Geometry: final body of the model. Coordinates: model frame, mm. Face numbers are marked on the shaded views. A direction names the side the tool comes from. Round coordinates to 2 decimals unless told otherwise and drop trailing zeros. Write each loop counter-clockwise with the first axis right and the second up, starting at its lowest first coordinate (ties: lowest second). Pieces come first, ordered by that corner, then holes.
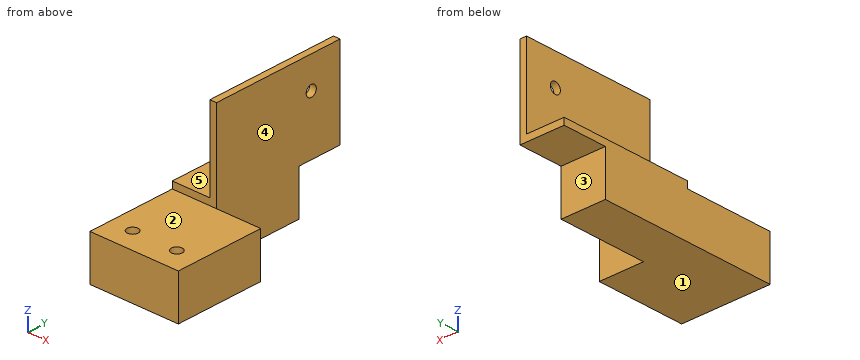
Autodesk Inventor part; units mm, degrees
ref_plane "YZ Plane" through (0, 0, 0) normal (1, 0, 0) x (0, 1, 0)
ref_plane "XZ Plane" through (0, 0, 0) normal (0, 1, 0) x (-1, 0, 0)
ref_plane "XY Plane" through (0, 0, 0) normal (0, 0, 1) x (1, 0, 0)
sketch "Náčrt1" plane through (0, 0, 0) normal (0, 0, 1) x (1, 0, 0)
  line L0 (-14, 0) -> (14, 0)
  line L1 (0, 28) -> (0, -28)
  line L2 (-10, 20) -> (10, 20)
  line L3 (10, 20) -> (10, -20)
  line L4 (10, -20) -> (-10, -20)
  line L5 (-10, -20) -> (-10, 20)
  point P0 (0, 0)
  dimension "d0" = 20
  dimension "d1" = 40
extrude "Vysunutí1" add sketch "Náčrt1" along normal mid plane 10
sketch "Náčrt2" plane through (0, 0, 5) normal (0, 0, 1) x (1, 0, 0)
  line L0 (-10, -20) -> (10, -20)
  line L1 (10, -20) -> (10, 20)
  line L2 (10, 20) -> (-10, 20)
  line L3 (-10, 20) -> (-10, -20)
  line L4 (10, -20) -> (10, 20)
  line L5 (0, 20) -> (10, 20)
  line L6 (10, 20) -> (10, 0)
  line L7 (10, 0) -> (0, 0)
  line L8 (0, 0) -> (0, 20)
  point P0 (0, 0)
extrude "Vysunutí2" cut sketch "Náčrt2" against normal through all contours L7 L8 L2 L1
sketch "Náčrt3" plane through (0, 0, 5) normal (0, 0, 1) x (1, 0, 0)
  line L0 (10, -20) -> (10, 0)
  line L1 (-10, -20) -> (10, -20)
  point P0 (0, 0)
  point P1 (-5, -15)
  point P2 (5, -15)
  dimension "d6" = 5
  dimension "d7" = 10
  dimension "d8" = 5
  dimension "d9" = 5
hole "Díra1" at (-5, -15, 5) at (5, -15, 5) direction (0, 0, -1) diameter 2.459 depth 5
sketch "Náčrt4" plane through (0, 0, 5) normal (0, 0, 1) x (1, 0, 0)
  line L0 (0, 0) -> (-10, 0)
  line L1 (-10, 0) -> (-10, 30)
  line L2 (-10, 30) -> (0, 30)
  line L3 (0, 30) -> (0, 0)
  dimension "d17" = 10
  dimension "d18" = 30
extrude "Vysunutí3" add sketch "Náčrt4" along normal blind 20
sketch "Náčrt5" plane through (-10, 30, 5) normal (0, 1, 0) x (1, 0, 0)
  line L0 (0, -20) -> (10, -20)
  line L1 (0, -20) -> (8.5, -20)
  line L2 (8.5, -20) -> (8.5, -1.5)
  line L3 (8.5, -1.5) -> (0, -1.5)
  line L4 (0, -1.5) -> (0, -20)
  point P0 (10, 5)
  dimension "d21" = 8.5
  dimension "d22" = 18.5
extrude "Vysunutí4" cut sketch "Náčrt5" against normal through all
sketch "Náčrt6" plane through (0, 0, -5) normal (1, 0, 0) x (0, 0, -1)
  line L0 (0, 20) -> (0, 0)
  line L1 (-10, 20) -> (0, 20)
  line L2 (-10, 20) -> (-10, 30)
  line L3 (-10, 30) -> (-30, 30)
  line L4 (-30, 0) -> (-30, 30)
  line L5 (-10, 0) -> (-30, 0)
  line L6 (-10, 0) -> (0, 0)
  point P0 (-5, 0)
  point P1 (-23, 23)
  dimension "d25" = 7
  dimension "d26" = 7
hole "Díra2" at (0, 23, 18) direction (-1, 0, 0) diameter 2.459 end through all
properties part number "x_bearing_tab" material "Hliník 6061"
1) Section B-B on x = -0.5. Output: boundary loops of the cut face in (y, z).
2) First-contact query: P1, Ø2.5, axis at x = -5.5, y = -15, coming from the +Z side; P2, Ø3, axis at x = -3.5, y = 24.5, coming from the -Z side; P3, Ø3, axis at y = 23, z = 18, coming from the +X side. Flat tips, straight axial feed; report the tip coordinate or a pass-through.
3) Reachability of the marked faces 1, 2, 3, 4 and 5 from +Z, -Z, +X, -X, +Y, -Y: full face, straight path, thin tool, end or side. Return the list, or none.
4) Line query: probe 1 along X at (y, z) = (-15, 3.7); probe 2 along Y at (x, z) = (-0.7, 18); probe 3 along Y at (x, z) = (5, 3.1). Output: solid intervals per line, ascending.
5) Section D-D on x = 5. Output: boundary loops of the cut face in (y, z).
6) Section C-C on z = 18. Output: boundary loops of the cut face in (x, y).
7) Section A-A on y = 23. Output: boundary loops of the cut face in (x, z).
Filled in:
1. outline: (-20, -5) - (20, -5) - (20, 5) - (30, 5) - (30, 25) - (0, 25) - (0, 5) - (-20, 5) - close; hole circle Ø2.46 at (23, 18)
2. P1: stops at z = 5
2. P2: stops at z = 5
2. P3: stops at x = 0
3. face 1: -Z, +X, -X, +Y, -Y
3. face 2: +Z, +X, -X, -Y
3. face 3: -Z, +X, -X, +Y
3. face 4: +Z, -Z, +X, +Y
3. face 5: +Z, -X, +Y, -Y
4. probe 1: x = -10 to -6.23, -3.77 to 3.77, 6.23 to 10
4. probe 2: y = 0 to 21.77, 24.23 to 30
4. probe 3: y = -20 to -16.23, -13.77 to 0
5. outline: (-20, -5) - (0, -5) - (0, 5) - (-13.77, 5) - (-13.77, 0) - (-16.23, 0) - (-16.23, 5) - (-20, 5) - close
6. outline: (-1.5, 0) - (0, 0) - (0, 21.77) - (-1.5, 21.77) - close; (-1.5, 24.23) - (0, 24.23) - (0, 30) - (-1.5, 30) - close
7. outline: (-10, 5) - (0, 5) - (0, 16.77) - (-1.5, 16.77) - (-1.5, 6.5) - (-10, 6.5) - close; (-1.5, 19.23) - (0, 19.23) - (0, 25) - (-1.5, 25) - close
